Read the model definition and answer for the solid it produces. Units are mm, in the model's axes. Face numbers are marked on the shaded views. A direction names the side the tool comes from. Give positions to 0.01 mm unless a question says otherwise; leave off trailing zeros. Write each loop counter-clockwise with the first axis right and the second up, starting at its lowest first coordinate (ties: lowest second). Pieces come first, ordered by that corner, then holes. Notation, with made-up numbers: (69.25, -20.5) -> (106.25, -20.5) arc R38 ccw to (106.25, 18.5) -> close; hole circle Ø10 at (68.5, -39.5). An arc over 180 degrees is marked (long way). Use a Markdown table: item, result.
from build123d import *

# Parameters (mm, degrees)
SKETCH2_W           = 60
SKETCH2_H           = 28
BOSS_EXTRUDE1_DEPTH = 30
SKETCH3_R           = 6
CUT_EXTRUDE1_DEPTH  = 47
SKETCH4_W           = 48
SKETCH4_H           = 20
BOSS_EXTRUDE2_DEPTH = 8
SKETCH5_W           = 36
SKETCH5_H           = 20
BOSS_EXTRUDE3_DEPTH = 12
SKETCH6_W           = 20
SKETCH6_H           = 20
BOSS_EXTRUDE4_DEPTH = 25


with BuildPart() as part:
    # Sketch2 → Boss-Extrude1 (new body)
    with BuildSketch(Plane(origin=(0, 0, 0), x_dir=(1, 0, 0), z_dir=(0, 1, 0))):
        Rectangle(SKETCH2_W, SKETCH2_H)
    extrude(amount=BOSS_EXTRUDE1_DEPTH)

    # Sketch3 → Cut-Extrude1 (cut)
    with BuildSketch(Plane.XY.offset(14)):
        with Locations((14, 16)):
            Circle(SKETCH3_R)
    extrude(amount=-CUT_EXTRUDE1_DEPTH, mode=Mode.SUBTRACT)

    # Sketch4 → Boss-Extrude2 (add)
    with BuildSketch(Plane(origin=(0, 30, 0), x_dir=(1, 0, 0), z_dir=(0, 1, 0))):
        with Locations((-6, 4)):
            Rectangle(SKETCH4_W, SKETCH4_H)
    extrude(amount=BOSS_EXTRUDE2_DEPTH)

    # Sketch5 → Boss-Extrude3 (add)
    with BuildSketch(Plane(origin=(0, 38, 0), x_dir=(1, 0, 0), z_dir=(0, 1, 0))):
        with Locations((-12, 4)):
            Rectangle(SKETCH5_W, SKETCH5_H)
    extrude(amount=BOSS_EXTRUDE3_DEPTH)

    # Sketch6 → Boss-Extrude4 (add)
    with BuildSketch(Plane(origin=(0, 50, 0), x_dir=(1, 0, 0), z_dir=(0, 1, 0))):
        with Locations((-20, 4)):
            Rectangle(SKETCH6_W, SKETCH6_H)
    extrude(amount=BOSS_EXTRUDE4_DEPTH)


solid = part.part
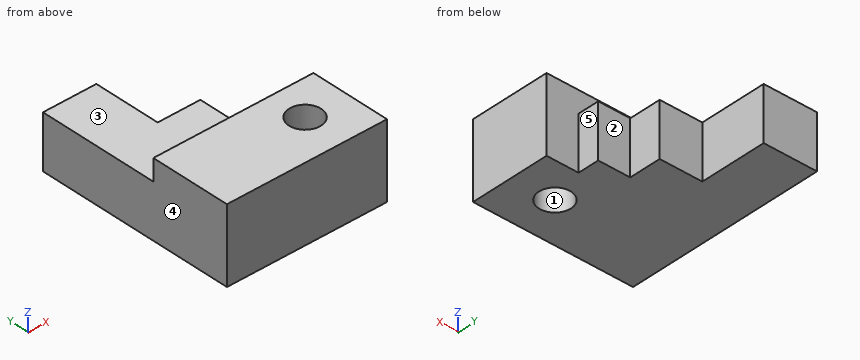
Item 1: For a pull along Y with two mould halves and no side action, classify the marked faces 1, 2 and 3 as +Y half, -Y half, draft (parallel to the pull), parting line (faces both ways), or undercut.
Return value:
| item | result |
|---|---|
| face 1 | undercut |
| face 2 | +Y half |
| face 3 | draft |
Item 2: A cutting plane is placed at C-C (x = 14). Give the vertices of the cut face in (y, z).
Return value:
| item | result |
|---|---|
| outline | (0, -14) -> (10, -14) -> (10, 14) -> (0, 14) -> close; (22, -14) -> (38, -14) -> (38, 6) -> (30, 6) -> (30, 14) -> (22, 14) -> close |
Item 3: A cutting plane is placed at B-B (z = 3.75). Give the vertices of the cut face in (x, y), then the cut area to 3 significant figures.
Return value:
| item | result |
|---|---|
| outline | (-30, 0) -> (30, 0) -> (30, 30) -> (18, 30) -> (18, 38) -> (6, 38) -> (6, 50) -> (-10, 50) -> (-10, 75) -> (-30, 75) -> close; hole circle Ø12 at (14, 16) |
| area | 3,000 mm^2 |
Item 4: Each of these flat-tipped pins is pushed along its axis until it touches: P1, Ø22.5, axis at x = -5.5, y = 47, coming from the +Z side; P2, Ø4, axis at y = 41, z = -4, coming from the +X side; P3, Ø10, axis at y = 38, z = -9.5, coming from the +X side. Where does it stop, or does it pass through?
Return value:
| item | result |
|---|---|
| P1 | z = 6 |
| P2 | x = 6 |
| P3 | x = 18 |
Item 5: A cutting plane is placed at A-A (y = 16). Give the vertices of the cut face in (x, z), then the cut area to 3 significant figures.
Return value:
| item | result |
|---|---|
| outline | (-30, -14) -> (8, -14) -> (8, 14) -> (-30, 14) -> close; (20, -14) -> (30, -14) -> (30, 14) -> (20, 14) -> close |
| area | 1,340 mm^2 |
Item 6: A tool of negligible diameter and unlimited length cuts with its end or side. For the marked faces 4 and 5, from which of +Z, -Z, +X, -X, +Y, -Y can it reach the whole face along a straight path? Write none if from no direction.
Return value:
| item | result |
|---|---|
| face 4 | +Z, -Z, -X, +Y, -Y |
| face 5 | +Z, -Z, +X, +Y |
Item 7: Straight lines are drawn through the part: line 1 along Y through (x, z) = (14, 4); line 2 along Z through (x, y) = (0, 38); line 3 along Y through (x, z) = (-21, 11.5). For each, find the intervals that lie inside material, in ascending order. Write a range as [from, to].
Return value:
| item | result |
|---|---|
| line 1 | [0, 10], [22, 38] |
| line 2 | [-14, 6] |
| line 3 | [0, 30] |
Item 8: A cutting plane is placed at D-D (x = -14.5). Give the vertices of the cut face in (y, z), then the cut area to 3 significant figures.
Return value:
| item | result |
|---|---|
| outline | (0, -14) -> (75, -14) -> (75, 6) -> (30, 6) -> (30, 14) -> (0, 14) -> close |
| area | 1,740 mm^2 |
